```python
from build123d import *

# Parameters (mm, degrees)
EXTRUDE_THIN4_DEPTH     = 6
CUT_EXTRUDE1_DEPTH      = 41
CUT_EXTRUDE1_DEPTH_BACK = 28
SKETCH3_R               = 1.5


with BuildPart() as part:
    # Sketch1 → Extrude-Thin4 (new body)
    with BuildSketch(Plane.XY):
        Polygon((-12.432700034, 0), (-2.432700034, 0), (-2.432700034, 25.5), (52.067299966, 25.5), (52.067299966, 0), (62.067299966, 0), (62.067299966, -3.550080031), (48.517219935, -3.550080031), (48.517219935, 21.949919969), (1.117379996, 21.949919969), (1.117379996, -3.550080031), (-12.432700034, -3.550080031), align=None)
    extrude(amount=EXTRUDE_THIN4_DEPTH)

    # Sketch3 → Cut-Extrude1 (cut, two sides: drawn at the far end of the back side and taken through both)
    with BuildSketch(Plane(origin=(0, 0, 0), x_dir=(1, 0, 0), z_dir=(0, 1, 0)).offset(-CUT_EXTRUDE1_DEPTH_BACK)):
        with Locations(Location((-7.639613875, -2.880964864, 0), (0, 0, 270))):
            Circle(SKETCH3_R)
        with Locations(Location((6.327175455, -2.880964864, 0), (0, 0, 270))):
            Circle(SKETCH3_R)
        with Locations(Location((42.196429871, -2.880964864, 0), (0, 0, 270))):
            Circle(SKETCH3_R)
        with Locations(Location((57.591640837, -2.880964864, 0), (0, 0, 180))):
            Circle(SKETCH3_R)
    extrude(amount=CUT_EXTRUDE1_DEPTH + CUT_EXTRUDE1_DEPTH_BACK, mode=Mode.SUBTRACT)


solid = part.part
```
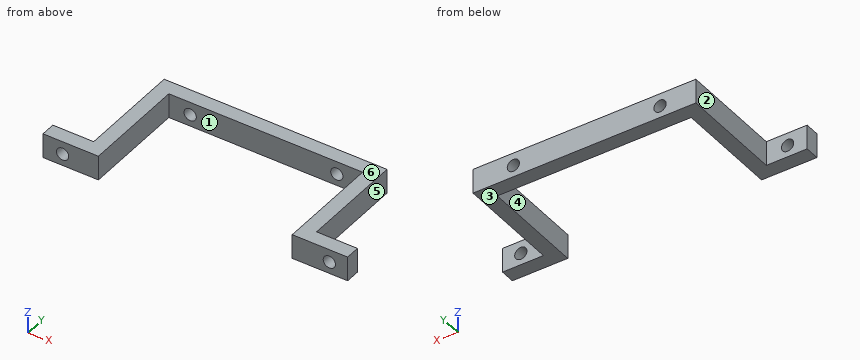
Read the model definition and answer for the solid it produces. Units are mm, in the model's axes. Face numbers are marked on the shaded views. A direction names the side the tool comes from. Coordinates: 2 decimals unless noted, no trailing zeros. Write each loop counter-clockwise with the first axis right and the second up, starting at its lowest first coordinate (ties: lowest second). Pieces come first, ordered by that corner, then holes. Notation, with made-up numbers: (-3, 32.5) -> (49, 32.5) arc R22 ccw to (49, 71.5) -> close; hole circle Ø2 at (26.25, 24.25). An arc over 180 degrees is marked (long way). Answer as a JSON object with one key per item and string values.
Q1. Determine the mould class of the marked faces 1, 2 and 3 for opening direction X: pulls with the +X half, pulls with the -X half, needs draft (parallel to the pull), parting line crosses it, or undercut.
The answers:
{"face 1": "undercut", "face 2": "pulls with the -X half", "face 3": "needs draft"}
Q2. The part is cut by section A-A on y = 20.25. Give the vertices of the cut face in (x, z).
The answers:
{"outline": "(-2.43, 0) -> (1.12, 0) -> (1.12, 6) -> (-2.43, 6) -> close; (48.52, 0) -> (52.07, 0) -> (52.07, 6) -> (48.52, 6) -> close"}
Q3. Flat-ended cylindrical pins translate along their axes: pin 1 Ø1.8 at (y, z) = (15.5, 1.5) entering from +X; pin 2 Ø1.8 at (x, z) = (22.5, 2) entering from -Y; pin 3 Ø1 at (y, z) = (11, 4) entering from -X. Find the tip coordinate at first contact, or state that the pin passes through.
The answers:
{"pin 1": "stops at x = 52.07", "pin 2": "stops at y = 21.95", "pin 3": "stops at x = -2.43"}
Q4. The part is cut by section B-B on z = 5.3. Give the vertices of the cut face in (x, y), then the cut area to 3 significant figures.
The answers:
{"outline": "(-12.43, -3.55) -> (1.12, -3.55) -> (1.12, 21.95) -> (48.52, 21.95) -> (48.52, -3.55) -> (62.07, -3.55) -> (62.07, 0) -> (52.07, 0) -> (52.07, 25.5) -> (-2.43, 25.5) -> (-2.43, 0) -> (-12.43, 0) -> close", "area": "446 mm2"}
Q5. The part is cut by section C-C on x = 20.5. Give the vertices of the cut face in (y, z).
The answers:
{"outline": "(21.95, 0) -> (25.5, 0) -> (25.5, 6) -> (21.95, 6) -> close"}
Q6. A tool of negligible diameter and unlimited length cuts with its end or side. For the marked faces 4, 5 and 6, from which of +Z, -Z, +X, -X, +Y, -Y can it reach the whole face along a straight path? Write none if from no direction.
The answers:
{"face 4": "+Z, -Z, -Y", "face 5": "+Z, -Z, +X, +Y", "face 6": "+Z, +X, -X, +Y, -Y"}
Q7. Consider line 1 (X direction, y = 17.75, z = 1.75); line 2 (Y direction, x = 37.5, z = 5.5); line 3 (Y direction, x = -3.5, z = 3.4). Determine where each line is inside the solid, lowest interval first. Write a range as [from, to].
The answers:
{"line 1": "x = [-2.43, 1.12], [48.52, 52.07]", "line 2": "y = [21.95, 25.5]", "line 3": "y = [-3.55, 0]"}
